Geometry check sheet. Reference: the model listing, model coordinates, mm. Round coordinates to 2 decimals unless told otherwise and drop trailing zeros. Order: outer loops, then holes, each group sorted by start corner. A loop starts at its lowest first (then second) coordinate and runs counter-clockwise, first axis right, second up. Notation, with made-up numbers: (-35, 2) - (6, 2) arc R21 ccw to (6, 40) - close; hole circle Ø5 at (64, 57.5). An arc over 180 degrees is marked (long way). Write each question's results on one line, items separated by ' | '.
```python
from build123d import *

# Parameters (mm, degrees)
SKETCH3_W           = 952.5
SKETCH3_H           = 577.85
BOSS_EXTRUDE2_DEPTH = 19.05
SKETCH4_R           = 76.2
CUT_EXTRUDE1_DEPTH  = 563.360531599


with BuildPart() as part:
    # Sketch3 → Boss-Extrude2 (new body)
    with BuildSketch(Plane(origin=(0, 711.2, 0), x_dir=(1, 0, 0), z_dir=(0, 1, 0))):
        with Locations((0, 9.525)):
            Rectangle(SKETCH3_W, SKETCH3_H)
    extrude(amount=-BOSS_EXTRUDE2_DEPTH)

    # Sketch4 → Cut-Extrude1 (cut, through all)
    with BuildSketch(Plane(origin=(0, 711.2, 0), x_dir=(1, 0, 0), z_dir=(0, 1, 0))):
        with Locations(Location((-349.25, 171.45, 0), (0, 0, 270))):
            Circle(SKETCH4_R)
    extrude(amount=-CUT_EXTRUDE1_DEPTH, mode=Mode.SUBTRACT)


solid = part.part
```
(1) Section check A-A (z = -171.45). Record the cut outline in (x, y).
Answers follow:
outline: (-476.25, 692.15) - (-425.45, 692.15) - (-425.45, 711.2) - (-476.25, 711.2) - close; (-273.05, 692.15) - (476.25, 692.15) - (476.25, 711.2) - (-273.05, 711.2) - close
(2) Material ranges on line 1 (X direction, y = 700.25, z = -171.45); line 2 (X direction, y = 710.25, z = -167), recorded low to high.
Answers follow:
line 1: -476.25 to -425.45, -273.05 to 476.25 | line 2: -476.25 to -425.32, -273.18 to 476.25
(3) Section check B-B (x = -349.25). Record the cut outline in (y, z).
Answers follow:
outline: (692.15, -298.45) - (711.2, -298.45) - (711.2, -247.65) - (692.15, -247.65) - close; (692.15, -95.25) - (711.2, -95.25) - (711.2, 279.4) - (692.15, 279.4) - close
(4) Section check C-C (y = 700.5). Record the cut outline in (x, z).
Answers follow:
outline: (-476.25, -298.45) - (476.25, -298.45) - (476.25, 279.4) - (-476.25, 279.4) - close; hole circle Ø152.4 at (-349.25, -171.45)
(5) Draft check along Z on faces 1 (the face through (-7, 711.2, -14)), 2 (the face through (-423.638, 701.808, -187.969)), 3 (the face through (-7, 702, -298.45)). Enter one of: released by +Z, released by -Z, zero draft, split by the parting line, or undercut.
Answers follow:
face 1: zero draft | face 2: undercut | face 3: released by -Z
